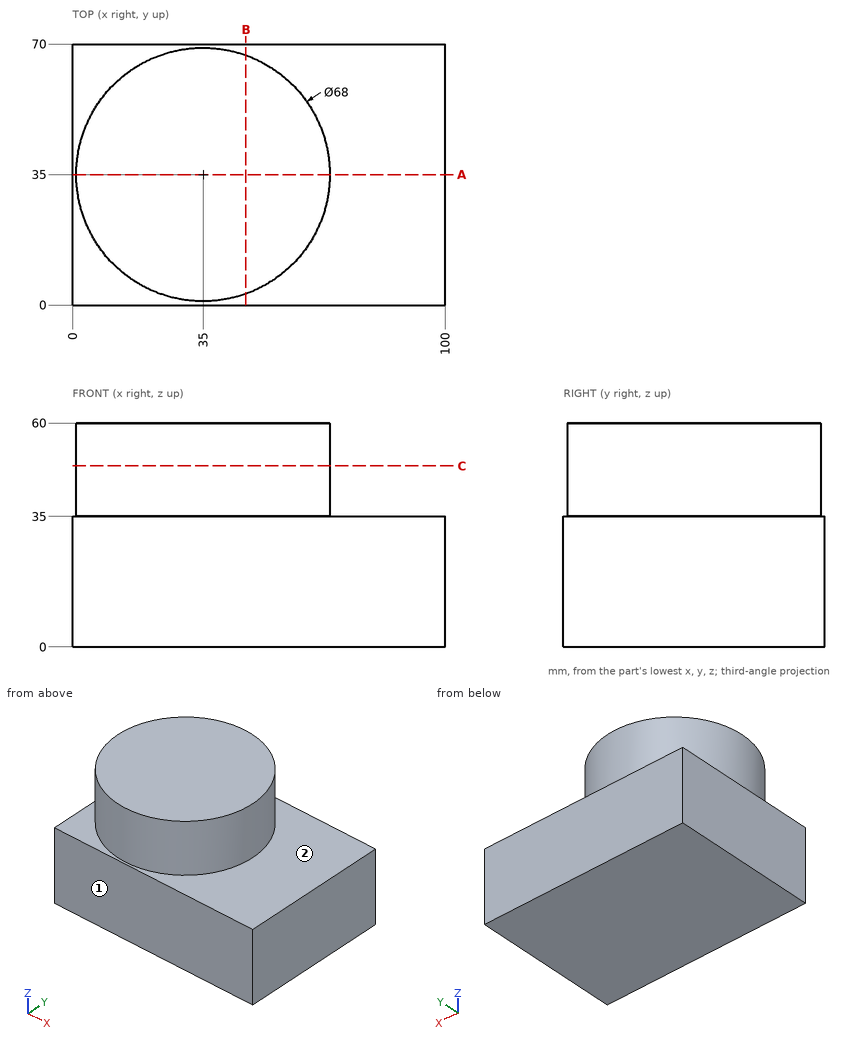
Answer from the drawing. Dimensions are ordinates in mm from the lowest x, y and z of the part. A direction names the side the tool comes from. Round coordinates to 2 decimals unless told otherwise and drop trailing zeros. Order: outer loops, then holes, each group sorted by start corner. A loop starts at its lowest first (then second) coordinate and runs counter-clockwise, first axis right, second up.
1) The part is cut by section B-B on x = 46.5. Write down the section's boundary in (y, z), plus the area to 3 significant figures.
2) Straight lines are drawn through the part: L1, parallel to Y at x = 34, z = 42; L2, parallel to Z at x = 80, y = 46; L3, parallel to X at y = 4, z = 41.5. For each, find the intervals that lie inside material, in ascending order.
3) For the marked faces 1 and 2, determine the directions among +Z, -Z, +X, -X, +Y, -Y from which every point of the face is accessible in a straight line to the end or side of a thin tool.
4) Flat-ended cylindrical pins translate along their axes: pin 1 (1 mm diameter, centred on x = 10, z = 8.5, fed in from -Y); pin 2 (10 mm diameter, centred on x = 21, z = 44, fed in from +Y); pin 3 (1.5 mm diameter, centred on y = 51.5, z = 53.5, fed in from -X). Find the tip coordinate at first contact, or state that the pin passes through.
5) The part is cut by section A-A on y = 35. Write down the section's boundary in (x, z).
6) The part is cut by section C-C on z = 48.5. Write down the section's boundary in (x, y).
Resolved:
1. outline: (0, 0) - (70, 0) - (70, 35) - (67, 35) - (67, 60) - (3, 60) - (3, 35) - (0, 35) - close
1. area: 4,050 mm2
2. L1: y = 1.01 to 68.99
2. L2: z = 0 to 35
2. L3: x = 21.04 to 48.96
3. face 1: +Z, -Z, +X, -X, -Y
3. face 2: +Z
4. pin 1: stops at y = 0
4. pin 2: stops at y = 67.79
4. pin 3: stops at x = 4.87
5. outline: (0, 0) - (100, 0) - (100, 35) - (69, 35) - (69, 60) - (1, 60) - (1, 35) - (0, 35) - close
6. outline: circle Ø68 at (35, 35)
